```python
from build123d import *

# Parameters (mm, degrees)
SKETCH2_R               = 20
BOSS_EXTRUDE1_DEPTH     = 20
SKETCH3_R               = 63.245553203
SKETCH3_R_2             = 55
CUT_EXTRUDE1_DEPTH      = 101
CUT_EXTRUDE1_DEPTH_BACK = 10


with BuildPart() as part:
    # Sketch1 → Revolve1 (revolve)
    with BuildSketch(Plane(origin=(0, 0, 0), x_dir=(1, 0, 0), z_dir=(0, 1, 0))):
        Polygon((70, -560), (70, -510), (60, -510), (60, -40), (0, -40), (0, -60), (45, -60), (45, -480), (25, -480), (25, -560), align=None)
    revolve(axis=Axis((0, 0, 0), (0, 0, 1)))

    # Sketch2 → Boss-Extrude1 (add, symmetric)
    with BuildSketch(Plane(origin=(0, 0, 0), x_dir=(1, 0, 0), z_dir=(0, 1, 0))):
        with BuildLine():
            Line((60, -40), (60, 0))
            ThreePointArc((60, 0), (0, 60), (-60, 0))
            Line((-60, 0), (-60, -40))
            Line((-60, -40), (60, -40))
        make_face()
        Circle(SKETCH2_R, mode=Mode.SUBTRACT)
    extrude(amount=BOSS_EXTRUDE1_DEPTH, both=True)

    # Sketch3 → Cut-Extrude1 (cut, two sides)
    with BuildSketch(Plane(origin=(0, 0, 40), x_dir=(-1, 0, 0), z_dir=(0, 0, -1))) as cut_extrude1_sk:
        Circle(SKETCH3_R)
        Circle(SKETCH3_R_2, mode=Mode.SUBTRACT)
    extrude(amount=CUT_EXTRUDE1_DEPTH, mode=Mode.SUBTRACT)
    extrude(cut_extrude1_sk.sketch, amount=-CUT_EXTRUDE1_DEPTH_BACK, mode=Mode.SUBTRACT)


solid = part.part
```
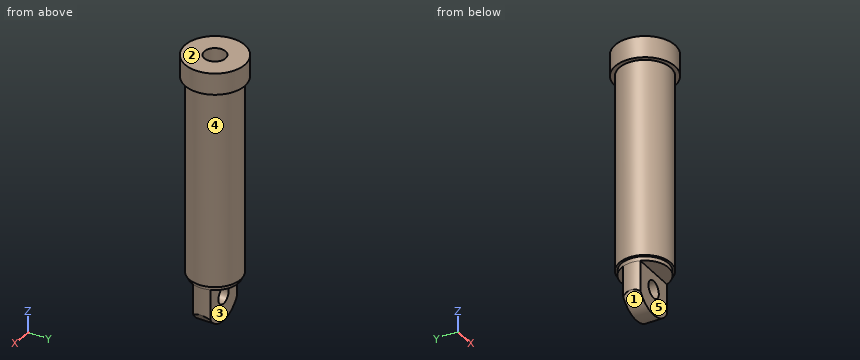
The listing builds one solid part. Answer for the finished solid, in the listing's coordinates (mm). Face numbers are marked on the shaded views. A direction names the side the tool comes from. Round coordinates to 2 decimals unless told otherwise and drop trailing zeros. Loops run counter-clockwise (first coordinate to the right, second up) from the corner with the lowest first, then second, coordinate; pieces in that order, holes last.
Q1. Section D-D, the plane z = 404 is taken. Determine the outline of the cut face in (x, y), then the cut area to 3 significant figures.
Q2. Section B-B, the plane y = 0 is taken. Determine the outline of the cut face in (x, z), then the cut area to 3 significant figures.
Q3. Given pin 1 Ø5 at (x, z) = (-48.5, 38.5) entering from +Y; pin 2 Ø12 at (y, z) = (27.5, 51.5) entering from -X; pin 3 Ø1.5 at (y, z) = (28.5, 284) entering from +X, each flat-ended and moving along its own axis, determine where each tip first touches the part or whether it passes through.
Q4. Section C-C, the plane x = 0 is taken. Determine the outline of the cut face in (y, z).
Q5. Which of the six approach directions +Z, -Z, +X, -X, +Y, -Y give full straight-line access (tool end or side, diameter ignored) to the marked faces 1, 2, 3, 4 and 5?
Q6. Find the intervals of material crossed by line 1 (Z direction, x = -28.5, y = 29); line 2 (Z direction, x = 0, y = -11); line 3 (X direction, y = 2.5, z = 123), in increasing order.
Q7. Section A-A, the plane z = 0 is taken. Determine the outline of the cut face in (x, y), then the cut area to 3 significant figures.
Completed:
1. outline: circle Ø120 at (0, 0); hole circle Ø90 at (0, 0)
1. area: 4,950 mm2
2. outline: (-70, 510) - (-60, 510) - (-60, 50) - (-55, 50) - (-55, -23.98) arc R60 ccw to (55, -23.98) - (55, 50) - (60, 50) - (60, 510) - (70, 510) - (70, 560) - (25, 560) - (25, 480) - (45, 480) - (45, 60) - (-45, 60) - (-45, 480) - (-25, 480) - (-25, 560) - (-70, 560) - close; hole circle Ø40 at (0, 0)
2. area: 30,100 mm2
3. pin 1: stops at y = 29.37
3. pin 2: stops at x = -56.02
3. pin 3: stops at x = 53.2
4. outline: (-70, 510) - (-60, 510) - (-60, 50) - (-55, 50) - (-55, 40) - (-20, 40) - (-20, 20) - (20, 20) - (20, 40) - (55, 40) - (55, 50) - (60, 50) - (60, 510) - (70, 510) - (70, 560) - (25, 560) - (25, 480) - (45, 480) - (45, 60) - (-45, 60) - (-45, 480) - (-25, 480) - (-25, 560) - (-70, 560) - close; (-20, -60) - (20, -60) - (20, -20) - (-20, -20) - close
5. face 1: -Z, +Y, -Y
5. face 2: +Z, +X, -X, +Y, -Y
5. face 3: -Z, +X, -X, +Y
5. face 4: -Z
5. face 5: -Z, +X, -X, -Y
6. line 1: z = 40 to 60, 480 to 560
6. line 2: z = -60 to -20, 20 to 60
6. line 3: x = -59.95 to -44.93, 44.93 to 59.95
7. outline: (-51.23, -20) - (-20, -20) - (-20, 20) - (-51.23, 20) arc R55 ccw to start; (20, -20) - (51.23, -20) arc R55 ccw to (51.23, 20) - (20, 20) - close
7. area: 2,700 mm2
